Input: part model. Units: mm. Frame: model coordinates. Face numbers are marked on the shaded views. A direction names the side the tool comes from. Give positions to 0.01 mm unless a question says otherwise; leave off trailing zeros. Write each loop counter-clockwise with the first axis right and the second up, starting at its lowest first coordinate (ties: lowest second). Pieces come first, ordered by that corner, then holes. Notation, with made-up numbers: (56, 12) - (79, 12) arc R20 ccw to (79, 20) - close; hole circle Ø4 at (46, -6.5). An arc over 180 degrees is marked (long way). Use a Markdown table: item, result. Add a question column.
1. Material intervals for probe 1 along Y at (x, z) = (3.5, 2.35); probe 2 along Y at (x, z) = (-20.5, 1.1); probe 3 along Y at (x, z) = (-11, 1), sorted ascending.
2. Section query A-A, the plane x = 8. Return loops of the section in (y, z), plus the area to 3 significant figures.
3. Section query B-B, the plane x = -9.5. Return loops of the section in (y, z).
4. Set-up query: the marked faces 4 and 5. Return all of +Z, -Z, +X, -X, +Y, -Y with unobstructed straight access to the full face (end or side cutting, diameter ignored); none if empty.
5. Pin query (flat end, axial travel): pin 1 (1.5 mm diameter, centred on x = 5.5, z = 1.5, fed in from +Y); pin 2 (1.3 mm diameter, centred on y = 0, z = 1.5, fed in from -X); pin 3 (1 mm diameter, centred on x = -0.5, z = 0.5, fed in from -Y). Return the tip coordinate at first contact, or that it passes through.
6. Mould query, pull axis X, two halves, no side actions, for the marked faces 1, 2 and 3. Classes: released by +X, released by -X, zero draft, split by the parting line, or undercut.
```python
from build123d import *

# Parameters (mm, degrees)
F1_DEPTH = 2.54


with BuildPart() as f1:
    # F0 (on Top) → F1 (new body)
    with BuildSketch(Plane.XY):
        Polygon((15.546987, -15.963222), (16.390529, -15.979688), (17.319008, -15.051209), (18.072152, -13.975608), (17.909457, -13.14774), (16.810267, -10.730381), (15.783584, -9.406071), (15.241934, -8.9693), (13.41697, -8.096944), (12.711619, -6.928926), (14.012052, -3.356017), (15.303169, -2.914654), (17.261912, -3.419454), (17.957592, -3.433034), (19.595327, -3.078493), (21.991203, -1.933234), (22.647978, -1.403629), (22.762419, -0.095559), (22.647978, 1.212511), (21.991203, 1.742116), (19.595327, 2.887375), (17.957592, 3.241916), (17.261912, 3.228336), (15.303169, 2.723536), (14.012052, 3.164899), (12.711619, 6.737808), (13.41697, 7.905826), (15.241934, 8.778182), (15.783584, 9.214953), (16.810267, 10.539263), (17.909457, 12.956622), (18.072152, 13.78449), (17.319008, 14.860091), (16.390529, 15.78857), (15.546987, 15.772104), (12.975481, 15.109383), (11.493009, 14.328262), (10.968816, 13.870685), (9.792812, 12.224929), (8.520056, 11.733119), (5.227245, 13.634224), (5.016787, 14.982369), (5.854051, 16.823696), (5.988228, 17.506449), (5.923463, 19.180868), (5.211642, 21.739218), (4.804131, 22.477979), (3.535806, 22.817826), (2.227736, 22.932268), (1.592129, 22.377436), (0.04823, 20.21683), (-0.585315, 18.665542), (-0.692745, 17.978073), (-0.535745, 15.96143), (-1.194603, 14.766569), (-4.93905, 14.106322), (-5.96684, 15.003781), (-6.509041, 16.952503), (-6.845121, 17.561769), (-7.97103, 18.802818), (-10.160792, 20.305079), (-10.94783, 20.60906), (-12.137873, 20.054134), (-13.213474, 19.30099), (-13.343738, 18.467404), (-13.137623, 15.819884), (-12.625797, 14.224294), (-12.266197, 13.628607), (-10.849655, 12.184687), (-10.586328, 10.845865), (-13.030342, 7.933202), (-14.394551, 7.960045), (-16.062515, 9.104332), (-16.711595, 9.355029), (-18.371823, 9.582008), (-21.014912, 9.325254), (-21.813214, 9.052219), (-22.36814, 7.862176), (-22.707986, 6.593851), (-22.271956, 5.871555), (-20.41227, 3.975926), (-18.994563, 3.082628), (-18.336193, 2.857452), (-16.322925, 2.66188), (-15.260626, 1.805546), (-15.260626, -1.996664), (-16.322925, -2.852998), (-18.336193, -3.04857), (-18.994563, -3.273746), (-20.41227, -4.167044), (-22.271956, -6.062673), (-22.707986, -6.784969), (-22.36814, -8.053294), (-21.813214, -9.243337), (-21.014912, -9.516372), (-18.371823, -9.773126), (-16.711595, -9.546147), (-16.062515, -9.29545), (-14.394551, -8.151163), (-13.030342, -8.12432), (-10.586328, -11.036983), (-10.849655, -12.375805), (-12.266197, -13.819725), (-12.625797, -14.415412), (-13.137623, -16.011002), (-13.343738, -18.658522), (-13.213474, -19.492108), (-12.137873, -20.245252), (-10.94783, -20.800178), (-10.160792, -20.496197), (-7.97103, -18.993936), (-6.845121, -17.752887), (-6.509041, -17.143621), (-5.96684, -15.194899), (-4.93905, -14.29744), (-1.194603, -14.957687), (-0.535745, -16.152548), (-0.692745, -18.169191), (-0.585315, -18.85666), (0.04823, -20.407948), (1.592129, -22.568554), (2.227736, -23.123386), (3.535806, -23.008944), (4.804131, -22.669097), (5.211642, -21.930336), (5.923463, -19.371986), (5.988228, -17.697567), (5.854051, -17.014814), (5.016787, -15.173487), (5.227245, -13.825342), (8.520056, -11.924237), (9.792812, -12.416047), (10.968816, -14.061803), (11.493009, -14.51938), (12.975481, -15.300501), align=None)
    extrude(amount=F1_DEPTH)


solid = f1.part
```
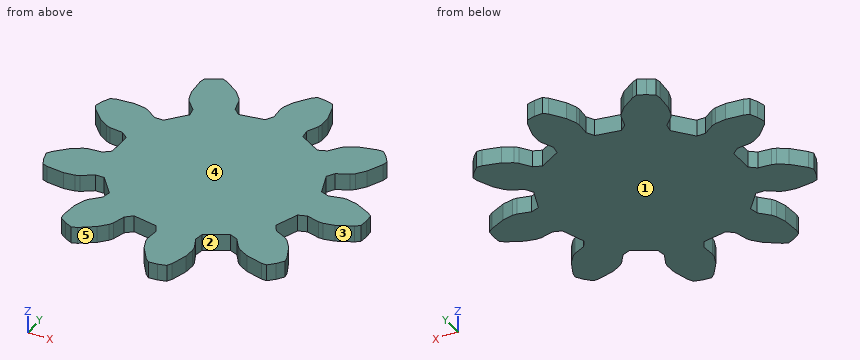
Result sheet:
| question | item | result |
|---|---|---|
| 1 | probe 1 | y = -23.01 to 22.82 |
| 1 | probe 2 | y = -9.57 to -4.26, 4.07 to 9.38 |
| 1 | probe 3 | y = -20.78 to -12.53, -10.54 to 10.35, 12.34 to 20.58 |
| 2 | outline | (-12.22, 0) - (12.03, 0) - (12.03, 2.54) - (-12.22, 2.54) - close |
| 2 | area | 61.6 mm² |
| 3 | outline | (-20.04, 0) - (19.85, 0) - (19.85, 2.54) - (-20.04, 2.54) - close |
| 4 | face 4 | +Z, +X, -X, +Y, -Y |
| 4 | face 5 | +Z, -Z, -Y |
| 5 | pin 1 | stops at y = 22.49 |
| 5 | pin 2 | stops at x = -15.26 |
| 5 | pin 3 | stops at y = -20.29 |
| 6 | face 1 | zero draft |
| 6 | face 2 | undercut |
| 6 | face 3 | released by +X |
